from build123d import *

# Parameters (mm, degrees)
F1_DEPTH     = 25.4
F2_R         = 2.38125
F3_DEPTH     = 28.576
F4_R         = 2.38125
F5_DEPTH     = 15.876
F6_T4_DEPTH  = 25.4
F6_S5_R      = 2.38125
F6_T6_DEPTH  = 15
F6_S7_R      = 2.38125
F6_T8_DEPTH  = 15
F6_T9_DEPTH  = 57.15
F6_T11_DEPTH = 34.925


# Not quite as in the source:
# - a fillet or chamfer that OpenCascade refuses, or shapes differently, is made with other operations: its cross-section is extruded or revolved along the edge and cut away or added


with BuildPart() as f1:
    # F0 (on Right) → F1 (new body)
    with BuildSketch(Plane.YZ):
        Polygon((0, 0), (12.7, 0), (12.7, 3.175), (-3.175, 3.175), (-3.175, -25.4), (0, -25.4), align=None)
    extrude(amount=F1_DEPTH)

    # F2 (on face) → F3 (cut, through all)
    with BuildSketch(Plane.XY.offset(3.175)):
        with Locations((6.35, 4.7625)):
            Circle(F2_R)
        with Locations((19.05, 4.7625)):
            Circle(F2_R)
    extrude(amount=-F3_DEPTH, mode=Mode.SUBTRACT)

    # F4 (on face) → F5 (cut, through all)
    with BuildSketch(Plane.XZ.offset(3.175)):
        with BuildLine():
            Line((13.550738686, -19.05), (11.849261314, -19.05))
            ThreePointArc((11.849261314, -19.05), (4.706499047, -22.0086289925), (0, -15.8749999656))
            Line((0, -15.8749999656), (0, -25.4))
            Line((0, -25.4), (25.4, -25.4))
            Line((25.4, -25.4), (25.4, -15.875))
            ThreePointArc((25.4, -15.875), (20.6935009364, -22.0086289969), (13.550738686, -19.05))
        make_face()
        with Locations((19.05, -15.875)):
            Circle(F4_R)
        with Locations((6.35, -15.875)):
            Circle(F4_R)
    extrude(amount=-F5_DEPTH, mode=Mode.SUBTRACT)

    # F6: fillet of radius 6.35 on 4 edges, made by hand


with BuildPart() as f6_tool2:
    # F6_s3 → F6_t4 (new body)
    with BuildSketch(Plane.YZ):
        with BuildLine():
            ThreePointArc((6.35, 0), (1.8598719395, -1.8598719395), (0, -6.35))
            Line((0, -6.35), (0, 0))
            Line((0, 0), (6.35, 0))
        make_face()
    extrude(amount=F6_T4_DEPTH)

    # F6_s5 → F6_t6 (cut, symmetric)
    with BuildSketch(Plane.XY.offset(-3.2)):
        with Locations((19.05, 4.7625)):
            Circle(F6_S5_R)
    extrude(amount=F6_T6_DEPTH, both=True, mode=Mode.SUBTRACT)

    # F6_s7 → F6_t8 (cut, symmetric)
    with BuildSketch(Plane.XY.offset(-3.2)):
        with Locations((6.35, 4.7625)):
            Circle(F6_S7_R)
    extrude(amount=F6_T8_DEPTH, both=True, mode=Mode.SUBTRACT)


with BuildPart() as f1_1:
    add(f1.part)

    # F6_t1: union F6_tool2
    add(f6_tool2.part)

    # F6_s10 → F6_t9 (cut)
    with BuildSketch(Plane.YZ.offset(-15.875)):
        with BuildLine():
            ThreePointArc((3.175, 3.175), (-1.3151280605, 1.3151280605), (-3.175, -3.175))
            Line((-3.175, -3.175), (-3.175, 3.175))
            Line((-3.175, 3.175), (3.175, 3.175))
        make_face()
    extrude(amount=F6_T9_DEPTH, mode=Mode.SUBTRACT)

    # F6_s12 → F6_t11 (cut)
    with BuildSketch(Plane.XY.offset(-15.875)):
        with BuildLine():
            ThreePointArc((6.35, 12.7), (1.8598719395, 10.8401280605), (0, 6.35))
            Line((0, 6.35), (0, 12.7))
            Line((0, 12.7), (6.35, 12.7))
        make_face()
        with BuildLine():
            ThreePointArc((25.4, 6.35), (23.5401280605, 10.8401280605), (19.05, 12.7))
            Line((19.05, 12.7), (25.4, 12.7))
            Line((25.4, 12.7), (25.4, 6.35))
        make_face()
    extrude(amount=F6_T11_DEPTH, mode=Mode.SUBTRACT)


solid = f1_1.part
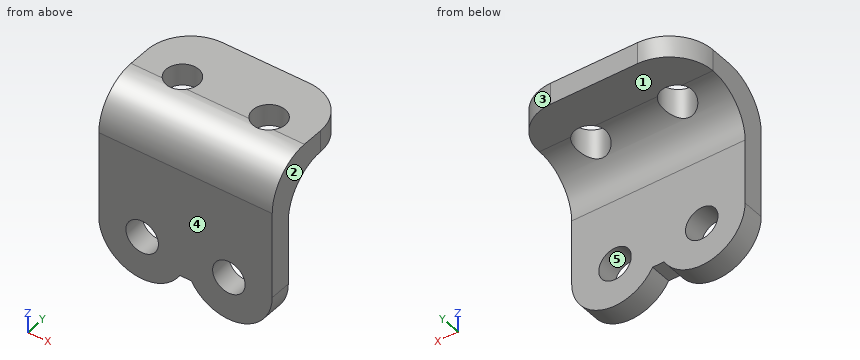
Verification items for the finished model (mm, model axes). Face numbers are marked on the shaded views. A direction names the side the tool comes from. Coordinates: 2 decimals unless noted, no trailing zeros. Order: outer loops, then holes, each group sorted by start corner. A loop starts at its lowest first (then second) coordinate and runs counter-clockwise, first axis right, second up. Notation, with made-up numbers: (50.25, 80.25) -> (71.25, 80.25) arc R26 cw to (71.25, 96.25) -> close; hole circle Ø7 at (89, -34). An arc over 180 degrees is marked (long way). Put each result on its own line as item: value. Start each with the question number.
1. Cross-section at B-B, the plane x = 17.75. Count the separate pieces of the cut face and the enclosed holes in it, then the cut area to 3 significant figures.
2. Cross-section at C-C, the plane z = 1. Record the boundary of the cut face in (x, y), then the cut area to 3 significant figures.
3. Cross-section at D-D, the plane z = -16.75. Record the boundary of the cut face in (x, y) (3 decimals).
4. Cross-section at A-A, the plane y = 5.25. Record the boundary of the cut face in (x, z) (3 decimals).
5. Material ranges on L1, parallel to Z at x = 7.75, y = 8.5 (3 decimals); L2, parallel to Y at x = 8.25, z = -11 (3 decimals); L3, parallel to Z at x = 19.05, y = -2.4 (3 decimals), recorded low to high. Write a range as [from, to].
6. Access from +Z, -Z, +X, -X, +Y, -Y to the whole of each face (thin tool, end or side, straight path). Record for the marked faces 1 and 2.
7. Mould release check, pull along X, two halves, no side actions. Record for the marked faces 3, 4 and 5: released by +X, released by -X, zero draft, split by the parting line, or undercut.
8. Go/stop test with flat-tipped pins: pin 1 Ø7.5 at (x, y) = (19.05, 4.76) entering from -Z; pin 2 Ø1.9 at (x, y) = (15, 10) entering from -Z; pin 3 Ø2 at (x, z) = (21, -14) entering from +Y; pin 4 Ø4 at (x, z) = (19.05, -15.875) entering from -Y. Record where each tip stops, or that it passes through.
Computed:
1. separate pieces: 3
1. enclosed holes: 0
1. area: 93.9 mm2
2. outline: (0, -1.61) -> (25.4, -1.61) -> (25.4, 6.35) arc R6.35 ccw to (19.05, 12.7) -> (6.35, 12.7) arc R6.35 ccw to (0, 6.35) -> close; hole circle Ø4.76 at (6.35, 4.76); hole circle Ø4.76 at (19.05, 4.76)
2. area: 311 mm2
3. outline: (0.061, -3.175) -> (4.135, -3.175) -> (4.135, 0) -> (0.061, 0) -> close; (8.565, -3.175) -> (16.835, -3.175) -> (16.835, 0) -> (8.565, 0) -> close; (21.265, -3.175) -> (25.339, -3.175) -> (25.339, 0) -> (21.265, 0) -> close
4. outline: (0, -0.096) -> (4.019, -0.096) -> (4.019, 3.175) -> (0, 3.175) -> close; (8.681, -0.096) -> (16.719, -0.096) -> (16.719, 3.175) -> (8.681, 3.175) -> close; (21.381, -0.096) -> (25.4, -0.096) -> (25.4, 3.175) -> (21.381, 3.175) -> close
5. L1: [0, 3.175]
5. L2: [-3.175, 0]
5. L3: [-22.225, -18.256], [-13.494, -0.135]
6. face 1: -Z, +X, -X, +Y
6. face 2: +Z, -Z, +X, +Y, -Y
7. face 3: released by +X
7. face 4: zero draft
7. face 5: undercut
8. pin 1: z = -2.91
8. pin 2: z = 0
8. pin 3: y = 0
8. pin 4: through
